from build123d import *

# Parameters (mm, degrees)
SKETCH_1_W        = 50
SKETCH_1_H        = 35
EXTRUDE_1_DEPTH   = 30
HOLE_WIZARD_341_D = 8.5
HOLE_WIZARD_446_D = 3.2
HOLE_WIZARD_600_D = 15
CHAMFER_1_SIZE    = 1
CHAMFER_1_SIZE_2  = 0.708203932


with BuildPart() as part:
    # 草图1 → 凸台-拉伸1 (new body)
    with BuildSketch(Plane.XY):
        Rectangle(SKETCH_1_W, SKETCH_1_H)
    extrude(amount=EXTRUDE_1_DEPTH)

    # Hole Wizard 341 (through all)
    with Locations(Plane.XY.offset(30)):
        with Locations((0, 0)):
            Hole(HOLE_WIZARD_341_D / 2)

    # Hole Wizard 446 (through all)
    with Locations(Plane.XY.offset(30)):
        with Locations((8, 0), (0, 8), (-8, 0), (0, -8)):
            Hole(HOLE_WIZARD_446_D / 2)

    # Hole Wizard 600 (through all)
    with Locations(Plane.XY.offset(30)):
        with Locations((20, 0), (-20, 0)):
            Hole(HOLE_WIZARD_600_D / 2)

    # 倒角1
    # the kernel refuses this chamfer: 1, 0.708203932 mm, written as the material it takes off along each edge
    with BuildSketch(Plane(origin=(-20, 0, 0), x_dir=(-0.8790200859122482, 0.4767847402789059, 0), z_dir=(-0.4767847402789059, -0.8790200859122482, 0))) as chamfer_1_piece_1:
        Polygon((7.5, -CHAMFER_1_SIZE), (7.5 + CHAMFER_1_SIZE, 0), (7.5, 0), align=None)
    revolve(axis=Axis((-20, 0, 0), (0, 0, -1)), revolution_arc=303.048763938, mode=Mode.SUBTRACT)
    with BuildSketch(Plane(origin=(-20, 0, 30), x_dir=(-0.879020085912248, 0.47678474027890627, 0), z_dir=(-0.47678474027890627, -0.879020085912248, 0))) as chamfer_1_piece_2:
        Polygon((7.5 + CHAMFER_1_SIZE, 0), (7.5, CHAMFER_1_SIZE), (7.5, 0), align=None)
    revolve(axis=Axis((-20, 0, 30), (0, 0, -1)), revolution_arc=303.048763938, mode=Mode.SUBTRACT)
    with BuildSketch(Plane(origin=(20, 0, 30), x_dir=(0.879020085912248, -0.4767847402789061, 0), z_dir=(0.4767847402789061, 0.879020085912248, 0))) as chamfer_1_piece_3:
        Polygon((7.5 + CHAMFER_1_SIZE, 0), (7.5, CHAMFER_1_SIZE), (7.5, 0), align=None)
    revolve(axis=Axis((20, 0, 30), (0, 0, -1)), revolution_arc=303.048763938, mode=Mode.SUBTRACT)
    with BuildSketch(Plane(origin=(20, 0, 0), x_dir=(0.8790200859122481, 0.476784740278906, 0), z_dir=(0.476784740278906, -0.8790200859122481, 0))) as chamfer_1_piece_4:
        Polygon((7.5, CHAMFER_1_SIZE), (7.5 + CHAMFER_1_SIZE, 0), (7.5, 0), align=None)
    revolve(axis=Axis((20, 0, 0), (0, 0, 1)), revolution_arc=303.048763938, mode=Mode.SUBTRACT)
    with BuildSketch(Plane(origin=(-25, 5.590169944, 32.778051389), x_dir=(0.7914486393779661, 0.611235675682274, 0), z_dir=(0, 0, -1)), Plane(origin=(25, -5.590169944, 32.778051389), x_dir=(-0.7914486393779661, -0.611235675682274, 0), z_dir=(0, 0, -1))) as chamfer_1_piece_5:
        with BuildLine():
            Line((1.080663788, 0), (CHAMFER_1_SIZE_2 * 0.611235676113, -CHAMFER_1_SIZE_2 * 0.791448639936))
            Line((CHAMFER_1_SIZE_2 * 0.611235676113, -CHAMFER_1_SIZE_2 * 0.791448639936), (0, 0))
            ThreePointArc((0, 0), (0.555522087, -0.019473843), (1.080663788, 0))
        make_face()
    extrude(amount=35.556102778, mode=Mode.SUBTRACT)
    with BuildSketch(Plane(origin=(-25, -5.590169944, 32.778051389), x_dir=(0.7914486393779665, -0.6112356756822735, 0), z_dir=(0, 0, -1))) as chamfer_1_piece_6:
        with BuildLine():
            Line((1.080663788, 0), (CHAMFER_1_SIZE_2 * 0.611235676113, CHAMFER_1_SIZE_2 * 0.791448639936))
            Line((CHAMFER_1_SIZE_2 * 0.611235676113, CHAMFER_1_SIZE_2 * 0.791448639936), (0, 0))
            ThreePointArc((0, 0), (0.555522087, 0.019473843), (1.080663788, 0))
        make_face()
    extrude(amount=35.556102778, mode=Mode.SUBTRACT)
    with BuildSketch(Plane(origin=(25, 5.590169944, 32.778051389), x_dir=(0, 1, 0), z_dir=(0, 0, -1))) as chamfer_1_piece_7:
        with BuildLine():
            Line((CHAMFER_1_SIZE_2, 0), (0.660540261, -0.855289885))
            ThreePointArc((0.660540261, -0.855289885), (0.354967464, -0.427764092), (0, 0))
            Line((0, 0), (CHAMFER_1_SIZE_2, 0))
        make_face()
    extrude(amount=35.556102778, mode=Mode.SUBTRACT)


solid = part.part
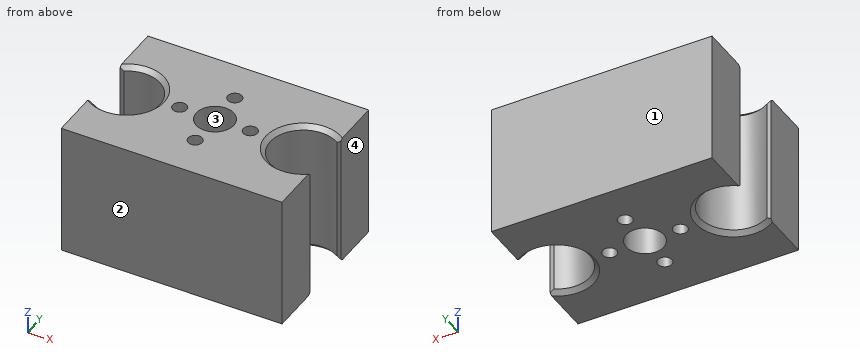
The listing builds one solid part. Answer for the finished solid, in the listing's coordinates (mm). Face numbers are marked on the shaded views. Round coordinates to 2 decimals unless told otherwise and drop trailing zeros. Loops run counter-clockwise (first coordinate to the right, second up) from the corner with the lowest first, then second, coordinate; pieces in that order, holes last. Notation, with made-up numbers: M 26,47 L 69,47 A23 cw 69,61 Z; hole C 32.5,31 d5. An arc over 180 degrees is marked long. Write each question's results on one line, items separated by ' | '. Start each with the question number.
1) Find section B-B on x = -20. Write down the section's boundary in (y, z), plus the area to 3 significant figures.
2) Straight lines are drawn through the part: probe 1 along Y at (x, z) = (0, 23.25); probe 2 along Y at (x, z) = (0.5, 6); probe 3 along Y at (x, z) = (-8, 12.5). For each, find the intervals that lie inside material, in ascending order.
3) Determine the mould class of the marked faces 1, 2, 3 and 4 for opening direction Y: pulls with the +Y half, pulls with the -Y half, needs draft (parallel to the pull), parting line crosses it, or undercut.
4) Each of these flat-tipped pins is pushed along its axis until it touches: pin 1 (6 mm diameter, centred on y = 6, z = 25, fed in from -X); pin 2 (1.5 mm diameter, centred on y = 4.5, z = 18.5, fed in from +X). Where does it stop, or does it pass through?
5) Find section A-A on y = 0. Write down the section's boundary in (x, z).
6) Find section D-D on x = -8. Write down the section's boundary in (y, z), plus the area to 3 significant figures.
7) Find section C-C on z = 23. Write down the section's boundary in (x, y), plus the area to 3 significant figures.
Final values:
1) outline: M -17.5,0 L -8.5,0 L -7.5,1 L -7.5,29 L -8.5,30 L -17.5,30 Z; M 7.5,1 L 8.5,0 L 17.5,0 L 17.5,30 L 8.5,30 L 7.5,29 Z | area: 598 mm²
2) probe 1: -17.5 to -9.6, -6.4 to -4.25, 4.25 to 6.4, 9.6 to 17.5 | probe 2: -17.5 to -9.52, -6.48 to -4.22, 4.22 to 6.48, 9.52 to 17.5 | probe 3: -17.5 to -1.6, 1.6 to 17.5
3) face 1: pulls with the +Y half | face 2: pulls with the -Y half | face 3: undercut | face 4: needs draft
4) pin 1: x = -25 | pin 2: x = 14.64
5) outline: M -12.5,1 L -11.5,0 L -9.6,0 L -9.6,30 L -11.5,30 L -12.5,29 Z; M -6.4,0 L -4.25,0 L -4.25,30 L -6.4,30 Z; M 4.25,0 L 6.4,0 L 6.4,30 L 4.25,30 Z; M 9.6,0 L 11.5,0 L 12.5,1 L 12.5,29 L 11.5,30 L 9.6,30 Z
6) outline: M -17.5,0 L -1.6,0 L -1.6,30 L -17.5,30 Z; M 1.6,0 L 17.5,0 L 17.5,30 L 1.6,30 Z | area: 954 mm²
7) outline: M -25,-17.5 L 25,-17.5 L 25,-6.3 L 24.14,-6.25 A7.5 cw long 24.14,6.25 L 25,6.3 L 25,17.5 L -25,17.5 L -25,6.3 L -24.14,6.25 A7.5 cw long -24.14,-6.25 L -25,-6.3 Z; hole C -8,0 d3.2; hole C 0,0 d8.5; hole C 0,-8 d3.2; hole C 0,8 d3.2; hole C 8,0 d3.2 | area: 1,350 mm²
